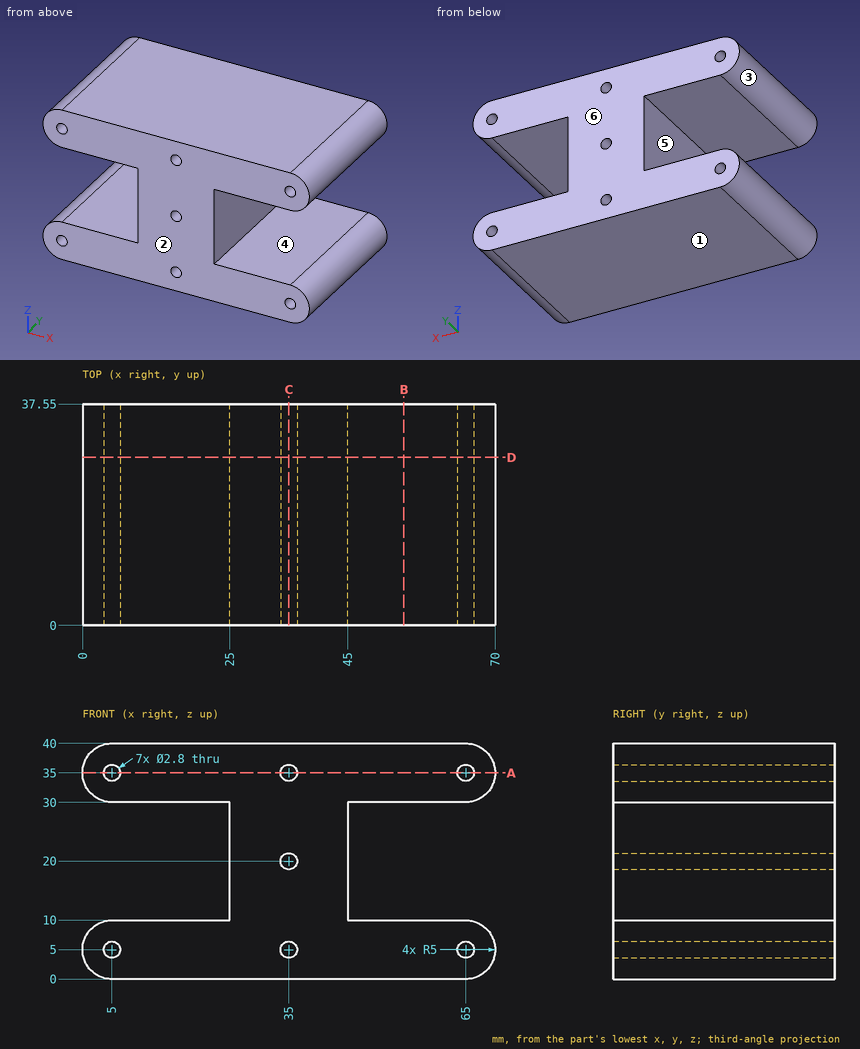
Geometry check sheet. Reference: drawing and pictorial views, mm from the part's lowest x, y, z. A direction names the side the tool comes from. Round coordinates to 2 decimals unless told otherwise and drop trailing zeros. Loops run counter-clockwise (first coordinate to the right, second up) from the corner with the lowest first, then second, coordinate; pieces in that order, holes last. Notation, with made-up numbers: (27.5, -19.75) - (64.5, -19.75) arc R18 cw to (64.5, 8.25) - close; hole circle Ø3 at (73.5, -15). An arc over 180 degrees is marked (long way). Write item = value, one per line. Start each with the question number.
Q1. Depth check by flat-ended pin: P1, Ø10, axis at x = 14.5, y = 16.5, coming from the -Z side; P2, Ø22, axis at y = 24.5, z = 22, coming from the +X side; P3, Ø1, axis at y = 7, z = 6, coming from the +X side; P4, Ø2, axis at x = 65, z = 35, coming from the -Y side. Enter the tip coordinate at first touch or a pass-through.
Q2. Section check D-D (y = 28.5). Record the boundary of the cut face in (x, z).
Q3. Thickness scan on L1, parallel to X at y = 14, z = 35; L2, parallel to Z at x = 61, y = 18.5; L3, parallel to Z at x = 65, y = 9. Record the ranges inside material, lowest first.
Q4. Section check A-A (z = 35). Record the boundary of the cut face in (x, y), plus the area to 3 significant figures.
Q5. Release check for a two-part mould opening along Z. For the marked faces 1, 2 and 3 record: pulls with the +Z half, pulls with the -Z half, needs draft (parallel to the pull), parting line crosses it, or undercut.
Q6. Access from +Z, -Z, +X, -X, +Y, -Y to the whole of each face (thin tool, end or side, straight path). Record for the marked faces 4, 5 and 6.
Q7. Section check B-B (x = 54.5). Record the boundary of the cut face in (y, z).
Q8. Section check C-C (x = 35). Record the boundary of the cut face in (y, z), plus the area to 3 significant figures.
Derived:
q1.P1 = 0
q1.P2 = 69.58
q1.P3 = 69.97
q1.P4 = through
q2.outline = (5, 0) - (65, 0) arc R5 ccw to (65, 10) - (45, 10) - (45, 30) - (65, 30) arc R5 ccw to (65, 40) - (5, 40) arc R5 ccw to (5, 30) - (25, 30) - (25, 10) - (5, 10) arc R5 ccw to start; hole circle Ø2.8 at (5, 5); hole circle Ø2.8 at (5, 35); hole circle Ø2.8 at (35, 5); hole circle Ø2.8 at (35, 20); hole circle Ø2.8 at (35, 35); hole circle Ø2.8 at (65, 5); hole circle Ø2.8 at (65, 35)
q3.L1 = 0 to 3.6, 6.4 to 33.6, 36.4 to 63.6, 66.4 to 70
q3.L2 = 0 to 10, 30 to 40
q3.L3 = 0 to 3.6, 6.4 to 10, 30 to 33.6, 36.4 to 40
q4.outline = (0, 0) - (3.6, 0) - (3.6, 37.55) - (0, 37.55) - close; (6.4, 0) - (33.6, 0) - (33.6, 37.55) - (6.4, 37.55) - close; (36.4, 0) - (63.6, 0) - (63.6, 37.55) - (36.4, 37.55) - close; (66.4, 0) - (70, 0) - (70, 37.55) - (66.4, 37.55) - close
q4.area = 2,310 mm^2
q5.face_1 = pulls with the -Z half
q5.face_2 = needs draft
q5.face_3 = undercut
q6.face_4 = +X, +Y, -Y
q6.face_5 = -X, +Y, -Y
q6.face_6 = +Z, -Z, +X, -X, +Y
q7.outline = (0, 0) - (37.55, 0) - (37.55, 10) - (0, 10) - close; (0, 30) - (37.55, 30) - (37.55, 40) - (0, 40) - close
q8.outline = (0, 0) - (37.55, 0) - (37.55, 3.6) - (0, 3.6) - close; (0, 6.4) - (37.55, 6.4) - (37.55, 18.6) - (0, 18.6) - close; (0, 21.4) - (37.55, 21.4) - (37.55, 33.6) - (0, 33.6) - close; (0, 36.4) - (37.55, 36.4) - (37.55, 40) - (0, 40) - close
q8.area = 1,190 mm^2
